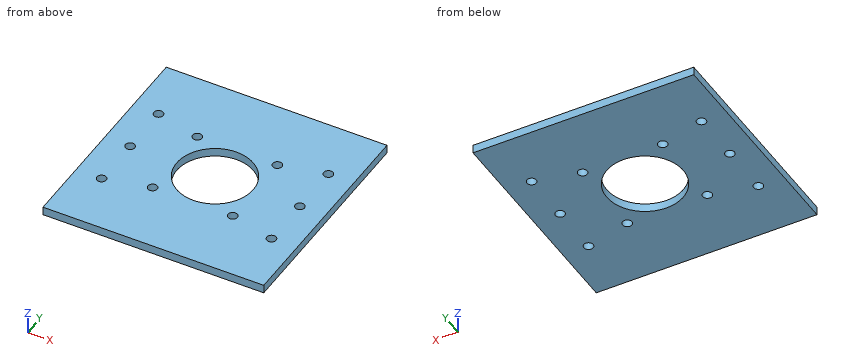
from build123d import *

# Parameters (mm, degrees)
SKETCH_1_W      = 130
SKETCH_1_H      = 130
SKETCH_1_R      = 22.5
SKETCH_1_R_2    = 2.75
EXTRUDE_1_DEPTH = 5


with BuildPart() as part:
    # 草图1 → 凸台-拉伸1 (new body)
    with BuildSketch(Plane.XY):
        Rectangle(SKETCH_1_W, SKETCH_1_H)
        Circle(SKETCH_1_R, mode=Mode.SUBTRACT)
        with Locations((-23.571404551, 23.571404551)):
            Circle(SKETCH_1_R_2, mode=Mode.SUBTRACT)
        with Locations((23.571404551, 23.571404551)):
            Circle(SKETCH_1_R_2, mode=Mode.SUBTRACT)
        with Locations((23.571404551, -23.571404551)):
            Circle(SKETCH_1_R_2, mode=Mode.SUBTRACT)
        with Locations((-23.571404551, -23.571404551)):
            Circle(SKETCH_1_R_2, mode=Mode.SUBTRACT)
        with Locations((-50, 30)):
            Circle(SKETCH_1_R_2, mode=Mode.SUBTRACT)
        with Locations((-50, 0)):
            Circle(SKETCH_1_R_2, mode=Mode.SUBTRACT)
        with Locations(Location((-50, -30, 0), (0, 0, 180))):
            Circle(SKETCH_1_R_2, mode=Mode.SUBTRACT)
        with Locations((50, -30)):
            Circle(SKETCH_1_R_2, mode=Mode.SUBTRACT)
        with Locations(Location((50, 0, 0), (0, 0, 180))):
            Circle(SKETCH_1_R_2, mode=Mode.SUBTRACT)
        with Locations(Location((50, 30, 0), (0, 0, 180))):
            Circle(SKETCH_1_R_2, mode=Mode.SUBTRACT)
    extrude(amount=EXTRUDE_1_DEPTH)


solid = part.part
For this review, take the finished solid that the model builds, in its own axes (mm). Give positions to 0.01 mm unless a question says otherwise; leave off trailing zeros. Loops run counter-clockwise (first coordinate to the right, second up) from the corner with the lowest first, then second, coordinate; pieces in that order, holes last. Notation, with made-up numbers: M 24.5,61 L 62.5,61 A32 cw 62.5,98 Z; hole C 27,-3 d8. An arc over 180 degrees is marked long. Put each result on its own line as item: value. Start each with the question number.
(1) Add section C-C, the plane x = 1. Write out the cut boundary in (y, z).
(2) Add section D-D, the plane x = 50. Write out the cut boundary in (y, z), then the cut area to 4 significant figures.
(3) Wall thickness on L1, parallel to Y at x = 50, z = 3.75; L2, parallel to Y at x = 25, z = 3.85; L3, parallel to Y at x = 51.5, z = 3.3: over which ranges is each line inside the solid? List them lowest first.
(4) For pin 1 (5 mm diameter, centred on x = -23.57, y = -23.57, fed in from -Z); pin 2 (7 mm diameter, centred on x = -50, y = -30, fed in from +Z), all flat-tipped, find the tip position at first contact; note any pin that passes through.
(5) Add section A-A, the plane y = 0. Write out the cut boundary in (x, z).
(6) Add section B-B, the plane y = 13.5. Write out the cut boundary in (x, z), then the cut area to 3 significant figures.
Result:
1. outline: M -65,0 L -22.48,0 L -22.48,5 L -65,5 Z; M 22.48,0 L 65,0 L 65,5 L 22.48,5 Z
2. outline: M -65,0 L -32.75,0 L -32.75,5 L -65,5 Z; M -27.25,0 L -2.75,0 L -2.75,5 L -27.25,5 Z; M 2.75,0 L 27.25,0 L 27.25,5 L 2.75,5 Z; M 32.75,0 L 65,0 L 65,5 L 32.75,5 Z
2. area: 567.5 mm^2
3. L1: y = -65 to -32.75, -27.25 to -2.75, 2.75 to 27.25, 32.75 to 65
3. L2: y = -65 to -25.92, -21.22 to 21.22, 25.92 to 65
3. L3: y = -65 to -32.3, -27.7 to -2.3, 2.3 to 27.7, 32.3 to 65
4. pin 1: passes through
4. pin 2: stops at z = 5
5. outline: M -65,0 L -52.75,0 L -52.75,5 L -65,5 Z; M -47.25,0 L -22.5,0 L -22.5,5 L -47.25,5 Z; M 22.5,0 L 47.25,0 L 47.25,5 L 22.5,5 Z; M 52.75,0 L 65,0 L 65,5 L 52.75,5 Z
6. outline: M -65,0 L -18,0 L -18,5 L -65,5 Z; M 18,0 L 65,0 L 65,5 L 18,5 Z
6. area: 470 mm^2
